Part print with two shaded views. Sizes in mm from the minimum x, y, z corner. A direction names the side the tool comes from. Round coordinates to 2 decimals unless told otherwise and drop trailing zeros. Write each loop counter-clockwise with the first axis right and the second up, starting at its lowest first coordinate (ties: lowest second). Pieces come first, ordered by that corner, then holes. Notation, with made-up numbers: (66, 61.5) -> (86, 61.5) arc R24 ccw to (86, 92.5) -> close; hole circle Ø3 at (81.25, 45.5). An arc over 180 degrees is marked (long way). Answer in a Markdown table with one row per item.
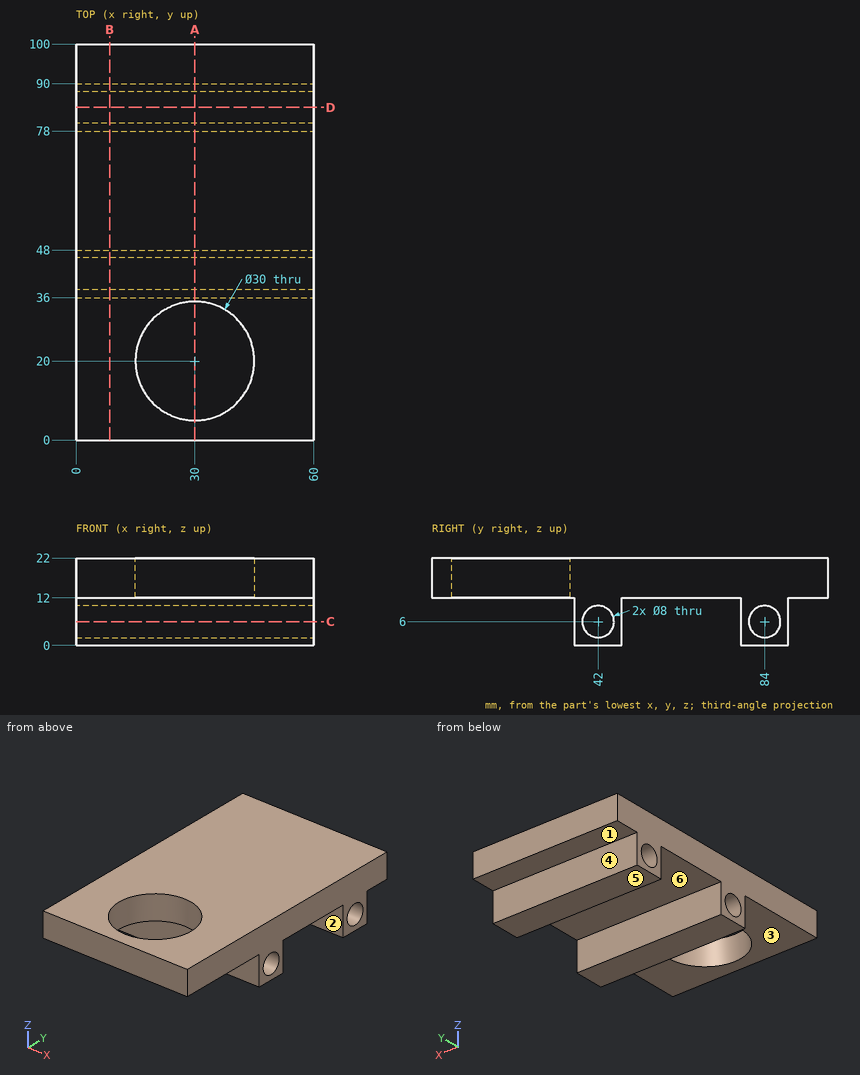
Q1. Wall check: line 1 (Y direction, x = 8, z = 6); line 2 (Y direction, x = 43.5, z = 11.25); line 3 (Y direction, x = 30, z = 19). Give the ranges that are in metal, low to high. Write a range as [from, to].
A:
| item | result |
|---|---|
| line 1 | [36, 38], [46, 48], [78, 80], [88, 90] |
| line 2 | [36, 48], [78, 90] |
| line 3 | [0, 5], [35, 100] |
Q2. Saw through at B-B on x = 8.5. Write the cut outline in (y, z), plus the area to 3 significant figures.
A:
| item | result |
|---|---|
| outline | (0, 12) -> (36, 12) -> (36, 0) -> (48, 0) -> (48, 12) -> (78, 12) -> (78, 0) -> (90, 0) -> (90, 12) -> (100, 12) -> (100, 22) -> (0, 22) -> close; hole circle Ø8 at (42, 6); hole circle Ø8 at (84, 6) |
| area | 1,190 mm² |
Q3. Saw through at D-D on y = 84. Write the cut outline in (x, z), plus the area to 3 significant figures.
A:
| item | result |
|---|---|
| outline | (0, 0) -> (60, 0) -> (60, 2) -> (0, 2) -> close; (0, 10) -> (60, 10) -> (60, 22) -> (0, 22) -> close |
| area | 840 mm² |
Q4. Saw through at A-A on x = 30. Write the cut outline in (y, z).
A:
| item | result |
|---|---|
| outline | (0, 12) -> (5, 12) -> (5, 22) -> (0, 22) -> close; (35, 12) -> (36, 12) -> (36, 0) -> (48, 0) -> (48, 12) -> (78, 12) -> (78, 0) -> (90, 0) -> (90, 12) -> (100, 12) -> (100, 22) -> (35, 22) -> close; hole circle Ø8 at (42, 6); hole circle Ø8 at (84, 6) |
Q5. Saw through at C-C on z = 6. Write the cut outline in (x, y).
A:
| item | result |
|---|---|
| outline | (0, 36) -> (60, 36) -> (60, 38) -> (0, 38) -> close; (0, 46) -> (60, 46) -> (60, 48) -> (0, 48) -> close; (0, 78) -> (60, 78) -> (60, 80) -> (0, 80) -> close; (0, 88) -> (60, 88) -> (60, 90) -> (0, 90) -> close |
Q6. Two-plate mould, pull along Y, no slides. Class the marked faces 4, 5 and 6: released by +Y, released by -Y, zero draft, split by the parting line, or undercut.
A:
| item | result |
|---|---|
| face 4 | released by +Y |
| face 5 | zero draft |
| face 6 | undercut |
Q7. Which spindle directions (+Z, -Z, +X, -X, +Y, -Y) get a long thin tool onto all of the face, cutting with end or side? Do the marked faces 1, 2 and 3. Say none if no direction does.
A:
| item | result |
|---|---|
| face 1 | -Z, +X, -X, +Y |
| face 2 | -Z, +X, -X |
| face 3 | -Z, +X, -X, -Y |
Q8. Drop flat-ended pins along their axis: P1, Ø3.5, axis at x = 42.5, z = 5, coming from the +Y side; P2, Ø6.5, axis at y = 42, z = 6, coming from the +X side; P3, Ø11, axis at x = 23, y = 97, coming from the -Z side; P4, Ø6, axis at x = 19, z = 7, coming from the -Y side. Give the stop position or say it passes through.
A:
| item | result |
|---|---|
| P1 | y = 90 |
| P2 | through |
| P3 | z = 12 |
| P4 | y = 36 |
